```python
from build123d import *

# Parameters (mm, degrees)
F0_W     = 76.2
F0_H     = 25.4
F1_DEPTH = 7.62
F3_DEPTH = 69.85
F4_W     = 0.860754
F4_H     = 25.4
F5_DEPTH = 5.08


with BuildPart() as f1:
    # F0 (on Top) → F1 (new body)
    with BuildSketch(Plane.XY):
        Rectangle(F0_W, F0_H)
    extrude(amount=F1_DEPTH)

    # F2 (on face) → F3 (cut)
    with BuildSketch(Plane(origin=(-38.1, 0, 0), x_dir=(0, -1, 0), z_dir=(-1, 0, 0))):
        Polygon((2.159, 7.62), (-2.159, 7.62), (-2.159, 5.349967), (0, 2.54), (2.159, 5.349967), align=None)
    extrude(amount=-F3_DEPTH, mode=Mode.SUBTRACT)

    # F4 (on face) → F5 (cut)
    with BuildSketch(Plane.XY.offset(7.62)):
        with Locations((-17.018, 0)):
            Rectangle(F4_W, F4_H)
    extrude(amount=-F5_DEPTH, mode=Mode.SUBTRACT)


solid = f1.part
```
Geometry: final body of the model. Coordinates: model frame, mm. A direction names the side the tool comes from. Round coordinates to 2 decimals unless told otherwise and drop trailing zeros. Order: outer loops, then holes, each group sorted by start corner. A loop starts at its lowest first (then second) coordinate and runs counter-clockwise, first axis right, second up. Notation, with made-up numbers: (89.25, 80) -> (96.25, 80) arc R29 ccw to (96.25, 101) -> close; hole circle Ø1 at (-9, 26.25). An arc over 180 degrees is marked (long way). Use one line per item in the form item = value.
(1) Access query for faces 4 (the face through (-17.448, -6, 5)), 5 (the face through (38.1, 0, 4)), 6 (the face through (-27.92, 1.09, 3.96)). Directions: +Z, -Z, +X, -X, +Y, -Y. A direction counts if a zero-diameter tool reaches every point of the face in a straight line with its end or side. Return the directions, or none.
Results list:
face_4 = +Z, +Y, -Y
face_5 = +Z, -Z, +X, +Y, -Y
face_6 = +Z, -X
(2) Section A-A on z = 6.5. Return loops of the section in (x, y), and give its area (3 significant figures).
Results list:
outline = (-38.1, -12.7) -> (-17.45, -12.7) -> (-17.45, -2.16) -> (-38.1, -2.16) -> close; (-38.1, 2.16) -> (-17.45, 2.16) -> (-17.45, 12.7) -> (-38.1, 12.7) -> close; (-16.59, -12.7) -> (38.1, -12.7) -> (38.1, 12.7) -> (-16.59, 12.7) -> (-16.59, 2.16) -> (31.75, 2.16) -> (31.75, -2.16) -> (-16.59, -2.16) -> close
area = 1,620 mm^2
(3) Draft query along X for faces 1 (the face through (31.75, 0, 6)), 2 (the face through (-1, -12.7, 4)), 3 (the face through (-17.448, 8, 5)). Return one class per face: pulls with the +X half, pulls with the -X half, needs draft (parallel to the pull), parting line crosses it, or undercut.
Results list:
face_1 = pulls with the -X half
face_2 = needs draft
face_3 = undercut
(4) Section B-B on x = -13. Return loops of the section in (y, z), and give its area (3 significant figures).
Results list:
outline = (-12.7, 0) -> (12.7, 0) -> (12.7, 7.62) -> (2.16, 7.62) -> (2.16, 5.35) -> (0, 2.54) -> (-2.16, 5.35) -> (-2.16, 7.62) -> (-12.7, 7.62) -> close
area = 178 mm^2
(5) Section C-C on z = 3.25. Return loops of the section in (x, y).
Results list:
outline = (-38.1, -12.7) -> (-17.45, -12.7) -> (-17.45, -0.55) -> (-38.1, -0.55) -> close; (-38.1, 0.55) -> (-17.45, 0.55) -> (-17.45, 12.7) -> (-38.1, 12.7) -> close; (-16.59, -12.7) -> (38.1, -12.7) -> (38.1, 12.7) -> (-16.59, 12.7) -> (-16.59, 0.55) -> (31.75, 0.55) -> (31.75, -0.55) -> (-16.59, -0.55) -> close
(6) First-contact query: pin 1 Ø4.5 at (y, z) = (0, 5) entering from -X. Flat tip, straight axial feed; report the tip coordinate or a pass-through.
Results list:
pin_1 = -38.1
(7) Ray query, probe 1 along Y at (x, z) = (-28, 6.25); probe 2 along X at (y, z) = (-10.5, 3.75); probe 3 along Y at (x, z) = (19, 4.75). Return the intervals inside material, ascending. Write a range as [from, to].
Results list:
probe_1 = [-12.7, -2.16], [2.16, 12.7]
probe_2 = [-38.1, -17.45], [-16.59, 38.1]
probe_3 = [-12.7, -1.7], [1.7, 12.7]
